```python
from build123d import *

# Parameters (mm, degrees)
SKETCH1_W           = 153
SKETCH1_H           = 20
BOSS_EXTRUDE1_DEPTH = 3
SKETCH2_W           = 3
SKETCH2_H           = 20
BOSS_EXTRUDE2_DEPTH = 17
SKETCH3_W           = 150
SKETCH3_H           = 3
BOSS_EXTRUDE3_DEPTH = 17
SKETCH4_R           = 1.6
SKETCH4_R_2         = 1.598435099
CUT_EXTRUDE1_DEPTH  = 10
SKETCH6_W           = 30
SKETCH6_H           = 17
BOSS_EXTRUDE4_DEPTH = 4
SKETCH7_R           = 2.1
CUT_EXTRUDE3_DEPTH  = 243.348358538
SKETCH8_R           = 4
CUT_EXTRUDE4_DEPTH  = 2.5
SKETCH9_W           = 30
SKETCH9_H           = 17
BOSS_EXTRUDE5_DEPTH = 4
SKETCH12_R          = 2.1
CUT_EXTRUDE7_DEPTH  = 243.348358538
SKETCH13_R          = 4
CUT_EXTRUDE8_DEPTH  = 2.5
CHAMFER9_SIZE       = 3
SKETCH15_W          = 3.1
SKETCH15_H          = 17
CUT_EXTRUDE10_DEPTH = 3


with BuildPart() as part:
    # Sketch1 → Boss-Extrude1 (new body)
    with BuildSketch(Plane.XY):
        with Locations((164.901588409, -32.175360178)):
            Rectangle(SKETCH1_W, SKETCH1_H)
    extrude(amount=BOSS_EXTRUDE1_DEPTH)

    # Sketch2 → Boss-Extrude2 (add)
    with BuildSketch(Plane(origin=(0, 0, 0), x_dir=(-1, 0, 0), z_dir=(0, 0, -1))):
        with Locations((-89.901588409, -32.175360178)):
            Rectangle(SKETCH2_W, SKETCH2_H)
    extrude(amount=BOSS_EXTRUDE2_DEPTH)

    # Sketch3 → Boss-Extrude3 (add)
    with BuildSketch(Plane(origin=(0, 0, 0), x_dir=(-1, 0, 0), z_dir=(0, 0, -1))):
        with Locations((-166.401588409, -40.675360178)):
            Rectangle(SKETCH3_W, SKETCH3_H)
    extrude(amount=BOSS_EXTRUDE3_DEPTH)

    # Sketch4 → Cut-Extrude1 (cut)
    with BuildSketch(Plane.ZY.offset(-88.401588409)):
        with Locations((-13, -27.175360178)):
            Circle(SKETCH4_R)
        with Locations((-4, -27.175360178)):
            Circle(SKETCH4_R)
        with Locations((-4, -35.175360178)):
            Circle(SKETCH4_R)
        with Locations((-13, -35.175360178)):
            Circle(SKETCH4_R_2)
    extrude(amount=-CUT_EXTRUDE1_DEPTH, mode=Mode.SUBTRACT)

    # Sketch6 → Boss-Extrude4 (add)
    with BuildSketch(Plane(origin=(0, -39.175360178, 0), x_dir=(1, 0, 0), z_dir=(0, 1, 0))):
        with Locations((226.401588409, 8.5)):
            Rectangle(SKETCH6_W, SKETCH6_H)
    extrude(amount=BOSS_EXTRUDE4_DEPTH)

    # Sketch7 → Cut-Extrude3 (cut, through all)
    with BuildSketch(Plane(origin=(0, -35.175360178, 0), x_dir=(1, 0, 0), z_dir=(0, 1, 0))):
        with Locations(Location((219.401588409, 8.5, 0), (0, 0, 270))):
            Circle(SKETCH7_R)
        with Locations(Location((233.401588409, 8.5, 0), (0, 0, 270))):
            Circle(SKETCH7_R)
    extrude(amount=-CUT_EXTRUDE3_DEPTH, mode=Mode.SUBTRACT)

    # Sketch8 → Cut-Extrude4 (cut)
    with BuildSketch(Plane.XZ.offset(42.175360178)):
        with Locations(Location((219.401588409, -8.5, 0), (0, 0, 270))):
            Circle(SKETCH8_R)
        with Locations(Location((233.401588409, -8.5, 0), (0, 0, 270))):
            Circle(SKETCH8_R)
    extrude(amount=-CUT_EXTRUDE4_DEPTH, mode=Mode.SUBTRACT)

    # Sketch9 → Boss-Extrude5 (add)
    with BuildSketch(Plane(origin=(0, -39.175360178, 0), x_dir=(1, 0, 0), z_dir=(0, 1, 0))):
        with Locations((156.401588409, 8.5)):
            Rectangle(SKETCH9_W, SKETCH9_H)
    extrude(amount=BOSS_EXTRUDE5_DEPTH)

    # Sketch12 → Cut-Extrude7 (cut, through all)
    with BuildSketch(Plane(origin=(0, -35.175360178, 0), x_dir=(1, 0, 0), z_dir=(0, 1, 0))):
        with Locations(Location((163.401588409, 8.5, 0), (0, 0, 270))):
            Circle(SKETCH12_R)
        with Locations(Location((149.401588409, 8.5, 0), (0, 0, 270))):
            Circle(SKETCH12_R)
    extrude(amount=-CUT_EXTRUDE7_DEPTH, mode=Mode.SUBTRACT)

    # Sketch13 → Cut-Extrude8 (cut)
    with BuildSketch(Plane.XZ.offset(42.175360178)):
        with Locations(Location((163.401588409, -8.5, 0), (0, 0, 270))):
            Circle(SKETCH13_R)
        with Locations(Location((149.401588409, -8.5, 0), (0, 0, 270))):
            Circle(SKETCH13_R)
    extrude(amount=-CUT_EXTRUDE8_DEPTH, mode=Mode.SUBTRACT)

    # Chamfer9
    chamfer9_edges = [part.edges().sort_by_distance(p)[0] for p in [
        (116.401588409, -39.175360178, 0),
        (191.401588409, -39.175360178, 0),
    ]]
    chamfer(chamfer9_edges, length=CHAMFER9_SIZE)

    # Sketch15 → Cut-Extrude10 (cut)
    with BuildSketch(Plane(origin=(0, -39.175360178, 0), x_dir=(1, 0, 0), z_dir=(0, 1, 0))):
        with Locations((209.851588409, 8.5)):
            Rectangle(SKETCH15_W, SKETCH15_H)
        with Locations((172.951588409, 8.5)):
            Rectangle(SKETCH15_W, SKETCH15_H)
        with Locations((139.851588409, 8.5)):
            Rectangle(SKETCH15_W, SKETCH15_H)
    extrude(amount=CUT_EXTRUDE10_DEPTH, mode=Mode.SUBTRACT)


solid = part.part
```
The model under review builds one solid part; all positions refer to its coordinate system, in mm. A direction names the side the tool comes from. Give positions to 0.01 mm unless a question says otherwise; leave off trailing zeros. Write each loop counter-clockwise with the first axis right and the second up, starting at its lowest first coordinate (ties: lowest second). Pieces come first, ordered by that corner, then holes. Notation, with made-up numbers: M -25,84.25 L 15,84.25 A22 ccw 15,109.25 Z; hole C 31.5,15.5 d11. An arc over 180 degrees is marked long. Write each question's results on one line, items separated by ' | '. Start each with the question number.
1. Mouldability with a two-part tool opening along X and no side actions: class faces 1 (the flat face through (226, -35.175, -9)), 2 (the cylindrical face through (221.484, -37.394, -8.773)) as released by +X, released by -X, zero draft, split by the parting line, or undercut.
2. For faces 3 (the cylindrical face through (89.88, -33.83, -12.14)), 4 (the flat face through (171.402, -37, -8)), 5 (the cylindrical face through (145.497, -40.943, -7.633)), 6 (the flat face through (156, -35.175, -9)), 7 (the cylindrical face through (89.88, -25.59, -4.21)), list the 3-axis set-ups (+Z, -Z, +X, -X, +Y, -Y) from which the entire face can be reached by the end or side of a thin tool; tool diameter is ignored.
3. Insertion check: pin 1 Ø2.5 at (x, z) = (220.5, -10.5) entering from -Y; pin 2 Ø2.5 at (x, z) = (233.4, -8.5) entering from +Y; pin 3 Ø5 at (y, z) = (-26, -8.5) entering from +X; pin 4 Ø4 at (x, z) = (138, -10) entering from +Y. Each pin has a flat end and moves straight along its axis. Give the tip position at first contact, or say it passes through.
4. We need section A-A (x = 189.5). Write out the cut boundary in (y, z).
5. For probe 1 along X at (y, z) = (-40.3, -8.5); probe 2 along X at (y, z) = (-36.75, -15); probe 3 along X at (y, z) = (-32.5, -3.75), list the stretches that pass through material, from the lowest coordinate up. Write a range as [from, to].
6. We need section B-B (z = -8.5). Count the separate pieces of the cut face and the enclosed holes in it, and give its area (3 significant figures).
Results found:
1) face 1: zero draft | face 2: undercut
2) face 3: -X | face 4: -Z, +Y | face 5: -Y | face 6: -Z, +X, +Y | face 7: +X, -X
3) pin 1: stops at y = -39.68 | pin 2: passes through | pin 3: stops at x = 91.4 | pin 4: stops at y = -39.18
4) outline: M -42.18,-17 L -39.18,-17 L -39.18,-3 L -36.18,0 L -22.18,0 L -22.18,3 L -42.18,3 Z
5) probe 1: x = [88.4, 145.4], [153.4, 159.4], [167.4, 215.4], [223.4, 229.4], [237.4, 241.4] | probe 2: x = [88.4, 91.4], [141.4, 171.4], [211.4, 241.4] | probe 3: x = [88.4, 91.4]
6) separate pieces: 5 | enclosed holes: 0 | area: 594 mm^2
